Read the model definition and answer for the solid it produces. Units are mm, in the model's axes. Face numbers are marked on the shaded views. A direction names the side the tool comes from. Coordinates: 2 decimals unless noted, no trailing zeros. Order: outer loops, then holes, each group sorted by start corner. A loop starts at its lowest first (then second) coordinate and runs counter-clockwise, first axis right, second up. Notation, with made-up numbers: M -13.75,26 L 22.25,26 A30 ccw 22.25,64 Z; hole C -11.75,67 d1. An arc over 180 degrees is marked long. One line per question, with ' | ' between items. Start each with the question number.
1) Consider probe 1 along Y at (x, z) = (0, -5.5); probe 2 along X at (y, z) = (1.5, -2.75); probe 3 along X at (y, z) = (-0.75, -5.25). Determine where each line is inside the solid, lowest interval first.
2) Find section C-C, the plane z = -10.25. Write down the section's boundary in (x, y), plus the area to 3 significant figures.
3) The mould has two halves that part along X. Classify the marked faces 4, 5 and 6: +X half, -X half, draft (parallel to the pull), parting line (faces both ways), or undercut.
4) Given P1, Ø1.5, axis at x = 3.5, z = -2.5, coming from the -Y side; P2, Ø6, axis at y = 5, z = -4, coming from the -X side; P3, Ø1, axis at x = 9.5, z = 2.5, coming from the +Y side, each flat-ended and moving along its own axis, determine where each tip first touches the part or whether it passes through.
5) A tool of negligible diameter and unlimited length cuts with its end or side. For the marked faces 1, 2 and 3, from which of +Z, -Z, +X, -X, +Y, -Y can it reach the whole face along a straight path? Write none if from no direction.
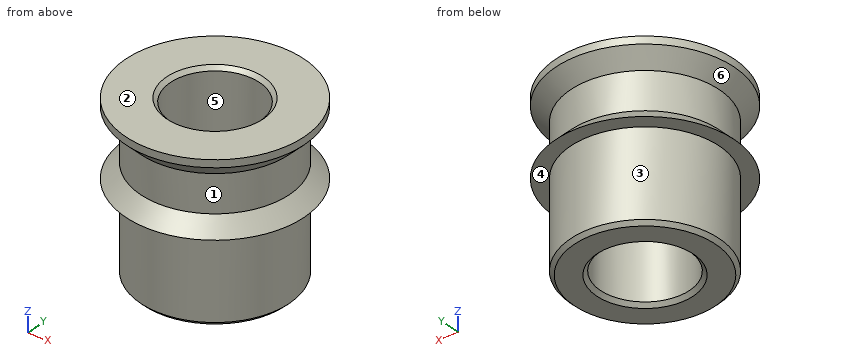
from build123d import *

# Parameters (mm, degrees)
F0_R     = 10
F0_R_2   = 6
F1_DEPTH = 12
F2_R     = 12
F2_R_2   = 6
F3_DEPTH = 2
F4_R     = 10
F4_R_2   = 6
F5_DEPTH = 5
F6_R     = 12
F6_R_2   = 6
F7_DEPTH = 3
F8_SIZE  = 1.99999
F9_SIZE  = 1.99999
F10_SIZE = 0.5


# Not quite as in the source:
# - a fillet or chamfer is up to 0.001 mm smaller than in the source, because OpenCascade refuses the exact size


with BuildPart() as f1:
    # F0 (on Top) → F1 (new body)
    with BuildSketch(Plane.XY):
        Circle(F0_R)
        Circle(F0_R_2, mode=Mode.SUBTRACT)
    extrude(amount=-F1_DEPTH)

    # F2 (on face) → F3 (join)
    with BuildSketch(Plane.XY):
        Circle(F2_R)
        Circle(F2_R_2, mode=Mode.SUBTRACT)
    extrude(amount=F3_DEPTH)

    # F4 (on face) → F5 (join)
    with BuildSketch(Plane.XY.offset(2)):
        Circle(F4_R)
        Circle(F4_R_2, mode=Mode.SUBTRACT)
    extrude(amount=F5_DEPTH)

    # F6 (on face) → F7 (join)
    with BuildSketch(Plane.XY.offset(7)):
        Circle(F6_R)
        Circle(F6_R_2, mode=Mode.SUBTRACT)
    extrude(amount=F7_DEPTH)

    # F8 (size 2 in the source; OpenCascade refuses exactly that, so slightly less here)
    f8_edges = [f1.edges().sort_by_distance(p)[0] for p in [
        (-12, 0, 2),
    ]]
    chamfer(f8_edges, length=F8_SIZE)

    # F9 (size 2 in the source; OpenCascade refuses exactly that, so slightly less here)
    f9_edges = [f1.edges().sort_by_distance(p)[0] for p in [
        (-12, 0, 7),
    ]]
    chamfer(f9_edges, length=F9_SIZE)

    # F10
    f10_edges = [f1.edges().sort_by_distance(p)[0] for p in [
        (-10, 0, -12),
        (-6, 0, -12),
        (-6, 0, 10),
    ]]
    chamfer(f10_edges, length=F10_SIZE)


solid = f1.part
Report:
1) probe 1: y = -10 to -6, 6 to 10 | probe 2: x = -9.89 to -5.81, 5.81 to 9.89 | probe 3: x = -9.97 to -5.95, 5.95 to 9.97
2) outline: C 0,0 d20; hole C 0,0 d12 | area: 201 mm^2
3) face 4: draft | face 5: undercut | face 6: parting line
4) P1: stops at y = -9.61 | P2: stops at x = -9.8 | P3: stops at y = 4.36
5) face 1: none | face 2: +Z, +X, -X, +Y, -Y | face 3: -Z
